Verification items for this drawing (mm, ordinates from the low corner). A direction names the side the tool comes from. Round coordinates to 2 decimals unless told otherwise and drop trailing zeros. Order: outer loops, then holes, each group sorted by start corner. A loop starts at its lowest first (then second) coordinate and runs counter-clockwise, first axis right, second up. Notation, with made-up numbers: M 87.5,4 L 132.5,4 A35 cw 132.5,36 Z; hole C 42,37.25 d11. An arc over 180 degrees is marked long. One line per item, written item: value. Start each with the question number.
(1) Cross-section at C-C, the plane y = 23.75. Enter the section's corners in (x, z), and give its area (3 significant figures).
(2) Cross-section at B-B, the plane y = 2.75. Enter the section's corners in (x, z), and give its area (3 significant figures).
(3) Access from +Z, -Z, +X, -X, +Y, -Y to the whole of each face (thin tool, end or side, straight path). Record for the marked faces 4, 5, 6, 7 and 8.
(4) Depth check by flat-ended pin: pin 1 Ø3 at (y, z) = (7, 1.5) entering from +X; pin 2 Ø5 at (x, y) = (17.5, 5.5) entering from +Z; pin 3 Ø3 at (x, z) = (28, 4.5) entering from -Y. Enter the tip coordinate at first touch or a pass-through.
(5) Cross-section at A-A, the plane z = 4.5. Enter the section's corners in (x, y), and give its area (3 significant figures).
(6) Thickness scan on L1, parallel to X at y = 2.5, z = 1.5; L2, parallel to Z at x = 4, y = 24.8; L3, parallel to X at y = 7.5, z = 5.25. Record the ranges inside material, lowest first.
(7) Release check for a two-part mould opening along Y. For the marked faces 1, 2 and 3 record: released by +Y, released by -Y, zero draft, split by the parting line, or undercut.
(8) Cross-section at D-D, the plane z = 6.25. Enter the section's corners in (x, y), and give its area (3 significant figures).
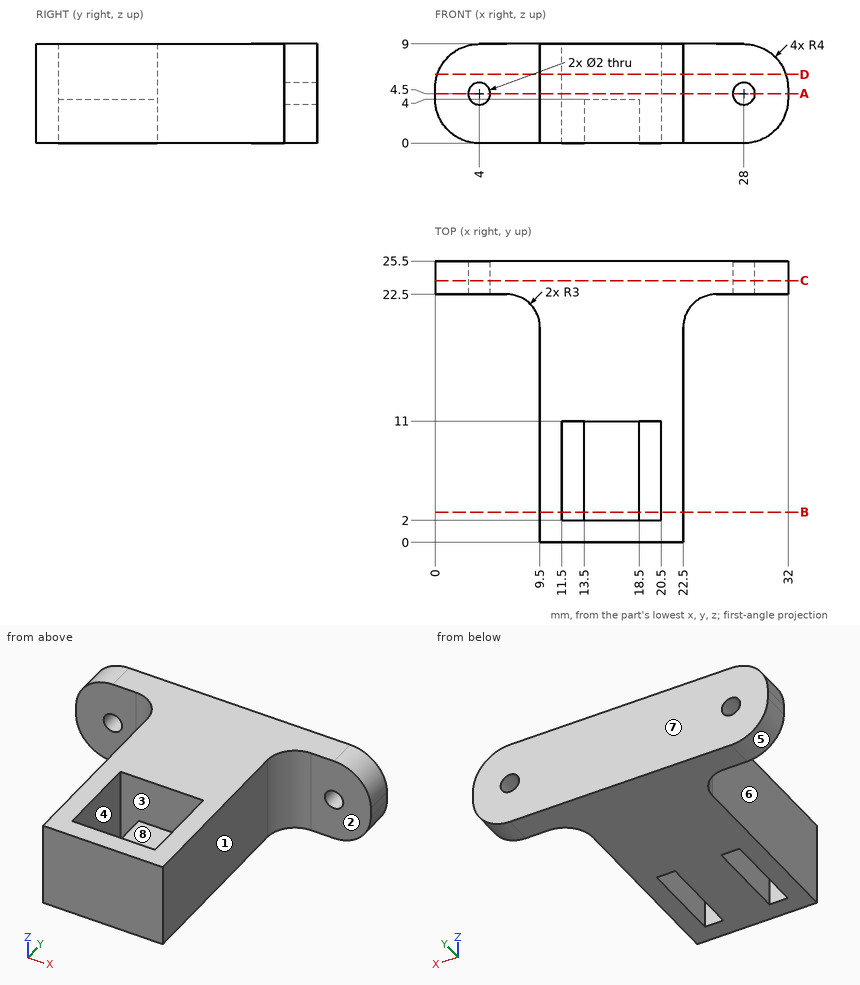
Values found:
1. outline: M 0,4 A4 ccw 4,0 L 28,0 A4 ccw 32,4 L 32,5 A4 ccw 28,9 L 4,9 A4 ccw 0,5 Z; hole C 4,4.5 d2; hole C 28,4.5 d2
1. area: 268 mm^2
2. outline: M 9.5,0 L 11.5,0 L 11.5,9 L 9.5,9 Z; M 13.5,0 L 18.5,0 L 18.5,4 L 13.5,4 Z; M 20.5,0 L 22.5,0 L 22.5,9 L 20.5,9 Z
2. area: 56.0 mm^2
3. face 4: +Z, -Z
3. face 5: -Z, -X, +Y, -Y
3. face 6: +Z, -Z, -X, -Y
3. face 7: +Z, -Z, +X, -X, +Y
3. face 8: +Z
4. pin 1: x = 22.5
4. pin 2: z = 4
4. pin 3: y = 22.5
5. outline: M 0,22.5 L 3,22.5 L 3,25.5 L 0,25.5 Z; M 5,22.5 L 6.5,22.5 A3 cw 9.5,19.5 L 9.5,0 L 22.5,0 L 22.5,19.5 A3 cw 25.5,22.5 L 27,22.5 L 27,25.5 L 5,25.5 Z; M 29,22.5 L 32,22.5 L 32,25.5 L 29,25.5 Z; hole M 11.5,2 L 20.5,2 L 20.5,11 L 11.5,11 Z
5. area: 299 mm^2
6. L1: 9.5 to 11.5, 13.5 to 18.5, 20.5 to 22.5
6. L2: 0 to 3.5, 5.5 to 9
6. L3: 9.5 to 11.5, 20.5 to 22.5
7. face 1: zero draft
7. face 2: released by -Y
7. face 3: undercut
8. outline: M 0.2,22.5 L 6.5,22.5 A3 cw 9.5,19.5 L 9.5,0 L 22.5,0 L 22.5,19.5 A3 cw 25.5,22.5 L 31.8,22.5 L 31.8,25.5 L 0.2,25.5 Z; hole M 11.5,2 L 20.5,2 L 20.5,11 L 11.5,11 Z
8. area: 310 mm^2
